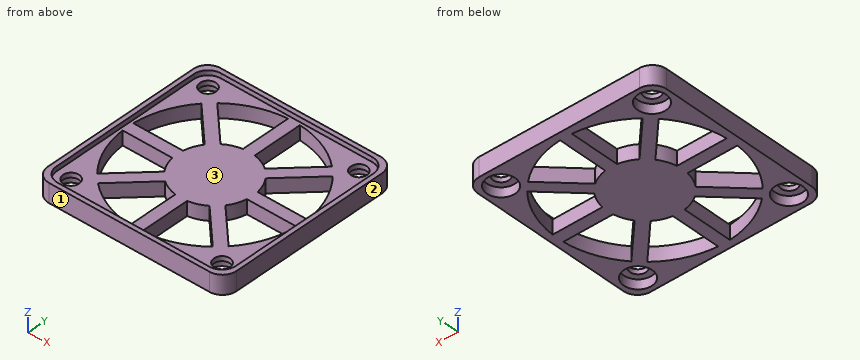
from build123d import *

# Parameters (mm, degrees)
F0_W     = 40
F0_H     = 40
F0_W_2   = 38.1
F0_H_2   = 38.1
F0_R     = 3
F0_R_2   = 18.5
F0_R_3   = 1.7
F1_DEPTH = 3
F0_R_4   = 8
F3_DEPTH = 3
F5_COUNT = 8
F6_DEPTH = 2
F7_DEPTH = 4
F8_R     = 3
F9_R     = 3


with BuildPart() as f1:
    # F0 (on Top) → F1 (new body)
    with BuildSketch(Plane.XY):
        Rectangle(F0_W, F0_H)
        Rectangle(F0_W_2, F0_H_2, mode=Mode.SUBTRACT)
        Rectangle(F0_W_2, F0_H_2)
        with Locations((-16, -16)):
            Circle(F0_R, mode=Mode.SUBTRACT)
        with Locations((16, -16)):
            Circle(F0_R, mode=Mode.SUBTRACT)
        with Locations((-16, 16)):
            Circle(F0_R, mode=Mode.SUBTRACT)
        Circle(F0_R_2, mode=Mode.SUBTRACT)
        with Locations((16, 16)):
            Circle(F0_R, mode=Mode.SUBTRACT)
        with Locations((-16, 16)):
            Circle(F0_R)
        with Locations((-16, 16)):
            Circle(F0_R_3, mode=Mode.SUBTRACT)
        with Locations((-16, -16)):
            Circle(F0_R)
        with Locations((-16, -16)):
            Circle(F0_R_3, mode=Mode.SUBTRACT)
        with Locations((16, -16)):
            Circle(F0_R)
        with Locations((16, -16)):
            Circle(F0_R_3, mode=Mode.SUBTRACT)
        with Locations((16, 16)):
            Circle(F0_R)
        with Locations((16, 16)):
            Circle(F0_R_3, mode=Mode.SUBTRACT)
    extrude(amount=F1_DEPTH)

    # F0 (on Top) → F6 (cut)
    with BuildSketch(Plane.XY):
        with Locations((16, -16)):
            Circle(F0_R)
        with Locations((16, -16)):
            Circle(F0_R_3, mode=Mode.SUBTRACT)
        with Locations((-16, -16)):
            Circle(F0_R)
        with Locations((-16, -16)):
            Circle(F0_R_3, mode=Mode.SUBTRACT)
        with Locations((-16, 16)):
            Circle(F0_R)
        with Locations((-16, 16)):
            Circle(F0_R_3, mode=Mode.SUBTRACT)
        with Locations((16, 16)):
            Circle(F0_R)
        with Locations((16, 16)):
            Circle(F0_R_3, mode=Mode.SUBTRACT)
    extrude(amount=F6_DEPTH, mode=Mode.SUBTRACT)



with BuildPart() as f1b:
    # F0 (on Top) → F1, piece 2 (new body)
    with BuildSketch(Plane.XY):
        Circle(F0_R_4)
    extrude(amount=F1_DEPTH)


with BuildPart() as f3:
    # F2 (on face) → F3 (new body)
    with BuildSketch(Plane.XY.offset(3)):
        with BuildLine():
            Line((1.25, 6), (1.25, 18.4577219613))
            ThreePointArc((1.25, 18.4577219613), (0, 18.5), (-1.25, 18.4577219613))
            Line((-1.25, 18.4577219613), (-1.25, 6))
            Line((-1.25, 6), (1.25, 6))
        make_face()
    extrude(amount=-F3_DEPTH)


with BuildPart() as f5_1:
    # F5: instance of F3
    add(f3.part.rotate(Axis((0, 0, 1.5), (0, 0, 1)), 1 * 360 / F5_COUNT))


with BuildPart() as f5_2:
    # F5: instance of F3
    add(f3.part.rotate(Axis((0, 0, 1.5), (0, 0, 1)), 2 * 360 / F5_COUNT))


with BuildPart() as f5_3:
    # F5: instance of F3
    add(f3.part.rotate(Axis((0, 0, 1.5), (0, 0, 1)), 3 * 360 / F5_COUNT))


with BuildPart() as f5_4:
    # F5: instance of F3
    add(f3.part.rotate(Axis((0, 0, 1.5), (0, 0, 1)), 4 * 360 / F5_COUNT))


with BuildPart() as f5_5:
    # F5: instance of F3
    add(f3.part.rotate(Axis((0, 0, 1.5), (0, 0, 1)), 5 * 360 / F5_COUNT))


with BuildPart() as f5_6:
    # F5: instance of F3
    add(f3.part.rotate(Axis((0, 0, 1.5), (0, 0, 1)), 6 * 360 / F5_COUNT))


with BuildPart() as f5_7:
    # F5: instance of F3
    add(f3.part.rotate(Axis((0, 0, 1.5), (0, 0, 1)), 7 * 360 / F5_COUNT))


with BuildPart() as f1_1:
    add(f1.part)

    add(f1b.part)  # F7 merges F1b

    add(f3.part)  # F7 merges F3

    add(f5_1.part)  # F7 merges F5_1

    add(f5_2.part)  # F7 merges F5_2

    add(f5_3.part)  # F7 merges F5_3

    add(f5_4.part)  # F7 merges F5_4

    add(f5_5.part)  # F7 merges F5_5

    add(f5_6.part)  # F7 merges F5_6

    add(f5_7.part)  # F7 merges F5_7
    # F0 (on Top) → F7 (join)
    with BuildSketch(Plane.XY):
        Rectangle(F0_W, F0_H)
        Rectangle(F0_W_2, F0_H_2, mode=Mode.SUBTRACT)
    extrude(amount=F7_DEPTH)

    # F8
    f8_edges = [f1_1.edges().sort_by_distance(p)[0] for p in [
        (-20, -20, 2),
        (20, -20, 2),
        (20, 20, 2),
        (-20, 20, 2),
    ]]
    fillet(f8_edges, radius=F8_R)

    # F9
    f9_edges = [f1_1.edges().sort_by_distance(p)[0] for p in [
        (-19.05, -19.05, 3.5),
        (-19.05, 19.05, 3.5),
        (19.05, 19.05, 3.5),
        (19.05, -19.05, 3.5),
    ]]
    fillet(f9_edges, radius=F9_R)


solid = f1_1.part
Verification items for the finished model (mm, model axes). Face numbers are marked on the shaded views. Coordinates: 2 decimals unless noted, no trailing zeros. Order: outer loops, then holes, each group sorted by start corner. A loop starts at its lowest first (then second) coordinate and runs counter-clockwise, first axis right, second up.
Item 1: Material ranges on L1, parallel to X at y = 9, z = 1.7; L2, parallel to Y at x = -16, z = 1; L3, parallel to Y at x = -4, z = 1.5, recorded low to high.
Filled in:
L1: x = -20 to -16.16, -10.77 to -7.23, -1.25 to 1.25, 7.23 to 10.77, 16.16 to 20
L2: y = -20 to -19, -13 to -9.29, -1.25 to 1.25, 9.29 to 13, 19 to 20
L3: y = -20 to -18.06, -6.93 to 6.93, 18.06 to 20
Item 2: Section check C-C, the plane y = -11. Enter the section's corners in (x, z), then the cut area to 3 significant figures.
Filled in:
outline: (-20, 0) - (-14.87, 0) - (-14.87, 3) - (-19.05, 3) - (-19.05, 4) - (-20, 4) - close; (-12.77, 0) - (-9.23, 0) - (-9.23, 3) - (-12.77, 3) - close; (-1.25, 0) - (1.25, 0) - (1.25, 3) - (-1.25, 3) - close; (9.23, 0) - (12.77, 0) - (12.77, 3) - (9.23, 3) - close; (14.87, 0) - (20, 0) - (20, 4) - (19.05, 4) - (19.05, 3) - (14.87, 3) - close
area: 61.4 mm2
Item 3: Section check D-D, the plane z = 0.9. Give the number of separate pieces and of enclosed holes in the cut face, then the cut area to 3 significant figures.
Filled in:
separate pieces: 1
enclosed holes: 12
area: 815 mm2
Item 4: Release check for a two-part mould opening along X. For the marked faces 1, 2 and 3 record: +X half, -X half, draft (parallel to the pull), parting line (faces both ways), or undercut.
Filled in:
face 1: draft
face 2: +X half
face 3: undercut
Item 5: Depth check by flat-ended pin: pin 1 (3 mm diameter, centred on x = -15, y = 14.5, fed in from -Z); pin 2 (3.5 mm diameter, centred on x = -16, y = 16, fed in from +Z); pin 3 (3.5 mm diameter, centred on x = 16, y = -16, fed in from -Z); pin 4 (1.5 mm diameter, centred on x = 5.5, y = 16, fed in from -Z). Enter the tip coordinate at first touch or a pass-through.
Filled in:
pin 1: stops at z = 0
pin 2: stops at z = 3
pin 3: stops at z = 2
pin 4: passes through
Item 6: Section check A-A, the plane x = 0.5. Enter the section's corners in (y, z), then the cut area to 3 significant figures.
Filled in:
outline: (-20, 0) - (20, 0) - (20, 4) - (19.05, 4) - (19.05, 3) - (-19.05, 3) - (-19.05, 4) - (-20, 4) - close
area: 122 mm2
Item 7: Section check B-B, the plane x = 10. Enter the section's corners in (y, z), then the cut area to 3 significant figures.
Filled in:
outline: (-20, 0) - (-15.56, 0) - (-15.56, 3) - (-19.05, 3) - (-19.05, 4) - (-20, 4) - close; (-11.77, 0) - (-8.23, 0) - (-8.23, 3) - (-11.77, 3) - close; (-1.25, 0) - (1.25, 0) - (1.25, 3) - (-1.25, 3) - close; (8.23, 0) - (11.77, 0) - (11.77, 3) - (8.23, 3) - close; (15.56, 0) - (20, 0) - (20, 4) - (19.05, 4) - (19.05, 3) - (15.56, 3) - close
area: 57.2 mm2
